from build123d import *

# Parameters (mm, degrees)
F1_DEPTH = 63.5
F0_W     = 20.569474
F0_H     = 19.05
F2_DEPTH = 25.4
F3_DEPTH = 7.9375


with BuildPart() as f1:
    # F0 (on Front) → F1 (new body, symmetric)
    with BuildSketch(Plane.XZ):
        Polygon((22.225, 9.525), (-41.275, 9.525), (-41.275, -9.525), (41.275, -9.525), (41.275, 9.525), align=None)
    extrude(amount=F1_DEPTH, both=True)

    # F0 (on Front) → F2 (join, symmetric)
    with BuildSketch(Plane.XZ):
        with BuildLine():
            Line((22.225, 27.0002), (22.225, 9.525))
            Line((22.225, 9.525), (41.275, 9.525))
            Line((41.275, 9.525), (41.275, 27.0002))
            ThreePointArc((41.275, 27.0002), (45.92468, 38.22552), (57.15, 42.8752))
            Line((57.15, 42.8752), (65.155526, 42.8752))
            Line((65.155526, 42.8752), (65.155526, 61.9252))
            Line((65.155526, 61.9252), (57.15, 61.9252))
            ThreePointArc((57.15, 61.9252), (32.454296, 51.695904), (22.225, 27.0002))
        make_face()
        with Locations((75.440263, 52.4002)):
            Rectangle(F0_W, F0_H)
    extrude(amount=F2_DEPTH, both=True)

    # F0 (on Front) → F3 (join, symmetric)
    with BuildSketch(Plane.XZ):
        with BuildLine():
            add(Edge.make_bspline(
                [(65.155526, 66.675), (13.582303, 67.183912), (-40.261839, 46.325367), (-41.275, 9.525)],
                knots=[0, 0, 0, 0, 120.803888, 120.803888, 120.803888, 120.803888], degree=3))
            Line((-41.275, 9.525), (22.225, 9.525))
            Line((22.225, 9.525), (22.225, 27.0002))
            ThreePointArc((22.225, 27.0002), (32.454296, 51.695904), (57.15, 61.9252))
            Line((57.15, 61.9252), (65.155526, 61.9252))
            Line((65.155526, 61.9252), (65.155526, 66.675))
        make_face()
    extrude(amount=F3_DEPTH, both=True)

    # F0 (on Front) → F4 (revolve)
    with BuildSketch(Plane.XZ):
        Polygon((115.955526, 66.675), (85.725, 66.675), (85.725, 61.9252), (85.725, 42.8752), (85.725, 38.1), (115.955526, 38.1), align=None)
    revolve(axis=Axis((85.725, 0, 40.4876), (0, 0, -1)))


solid = f1.part
CAD build for the part. Positions are in the model's coordinates, mm. A direction names the side the tool comes from. Round coordinates to 2 decimals unless told otherwise and drop trailing zeros. Write each loop counter-clockwise with the first axis right and the second up, starting at its lowest first coordinate (ties: lowest second). Pieces come first, ordered by that corner, then holes.
(1) Mould opens along X. For faces 1 (the face through (22.225, 17, 18)), 2 (the face through (-1, 63.5, 0)), 3 (the face through (60, 21, 42.875)) say: pulls with the +X half, pulls with the -X half, needs draft (parallel to the pull), parting line crosses it, or undercut.
(2) 3-axis set-ups, long thin cutter, end or side, ignore diameter. For faces 4 (the face through (32.73, 16.55, 51.97)), 5 (the face through (40, -25.4, 36)), 6 (the face through (85, 0, 66.675)), 7 (the face through (86, 0, 38.1)), 8 (the face through (-1, -63.5, 0)): which of +Z, -Z, +X, -X, +Y, -Y reach the whole face in a straight line?
(3) Slice it at C-C, the plane x = 85. Write the cut outline in (y, z) (3 decimals), and give its area (3 significant figures).
(4) Slice it at A-A, the plane y = -15.5. Write the cut outline in (x, z) (3 decimals), and give its area (3 significant figures).
(5) Drop flat-ended pins along their axis: P1, Ø17, axis at x = 13.5, z = 28, coming from the +Y side; P2, Ø5, axis at y = 44.5, z = 10, coming from the +X side (3 decimals); P3, Ø2, axis at x = 44.5, y = 3, coming from the -Z side. Give the stop position or say it passes through.
(6) Slice it at B-B, the plane z = -3.5. Write the cut outline in (x, y) (3 decimals), and give its area (3 significant figures).
(7) Probe line 1 along X through (y, z) = (-43.5, 6) (3 decimals); line 2 along Z through (x, y) = (92, 22) (3 decimals); line 3 along Y through (x, z) = (67, 58). List the from-to ranges inside material, lowest first.
From the geometry:
1. face 1: pulls with the -X half
1. face 2: needs draft
1. face 3: undercut
2. face 4: +Z, -X, +Y
2. face 5: +Z, -X, -Y
2. face 6: +Z, +X, -X, +Y, -Y
2. face 7: -Z, +X, +Y, -Y
2. face 8: +Z, -Z, +X, -X, -Y
3. outline: (-30.222, 38.1) - (30.222, 38.1) - (30.222, 66.675) - (-30.222, 66.675) - close
3. area: 1,730 mm2
4. outline: (-41.275, -9.525) - (41.275, -9.525) - (41.275, 27) arc R15.875 cw to (57.15, 42.875) - (59.771, 42.875) - (59.771, 38.1) - (111.679, 38.1) - (111.679, 66.675) - (59.771, 66.675) - (59.771, 61.925) - (57.15, 61.925) arc R34.925 ccw to (22.225, 27) - (22.225, 9.525) - (-41.275, 9.525) - close
4. area: 4,200 mm2
5. P1: stops at y = 7.94
5. P2: stops at x = 41.275
5. P3: stops at z = 35.11
6. outline: (-41.275, -63.5) - (41.275, -63.5) - (41.275, 63.5) - (-41.275, 63.5) - close
6. area: 10,500 mm2
7. line 1: x = -41.275 to 41.275
7. line 2: z = 38.1 to 66.675
7. line 3: y = -25.4 to 25.4
